The model under review builds one solid part; all positions refer to its coordinate system, in mm. Give positions to 0.01 mm unless a question says otherwise; leave off trailing zeros. Loops run counter-clockwise (first coordinate to the right, second up) from the corner with the lowest first, then second, coordinate; pieces in that order, holes last. Notation, with made-up numbers: (15.25, 22) - (69.25, 22) arc R13 ccw to (69.25, 47) - close; hole circle Ø3 at (47.25, 21). An arc over 180 degrees is marked (long way). Answer as a JSON object with one key per item and string values.
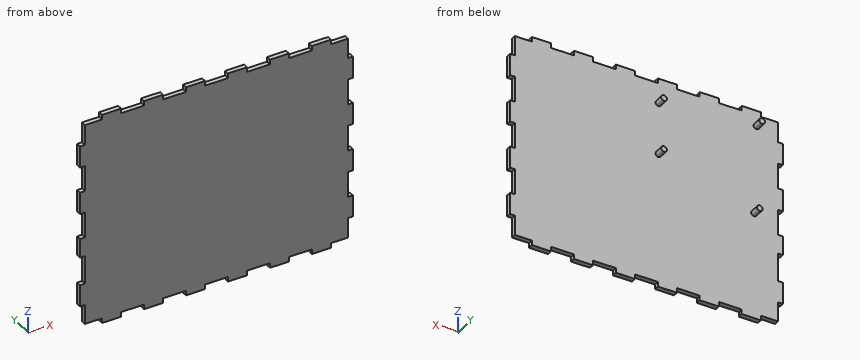
from build123d import *

# Parameters (mm, degrees)
SKETCH1_W           = 144.78
SKETCH1_H           = 114.3
BOSS_EXTRUDE1_DEPTH = 63.5
SKETCH2_W           = 144.78
SKETCH2_H           = 114.3
CUT_EXTRUDE1_DEPTH  = 60.96
SKETCH3_R           = 1.524
BOSS_EXTRUDE2_DEPTH = 5.08
SKETCH4_OUTSIDE_W   = 183.704
SKETCH4_OUTSIDE_H   = 153.224
CUT_EXTRUDE2_DEPTH  = 2.54
SKETCH6_OUTSIDE_W   = 183.704
SKETCH6_OUTSIDE_H   = 153.224
CUT_EXTRUDE4_DEPTH  = 2.54


with BuildPart() as part:
    # Sketch1 → Boss-Extrude1 (new body)
    with BuildSketch(Plane(origin=(0, 0, 0), x_dir=(1, 0, 0), z_dir=(0, 1, 0))):
        Rectangle(SKETCH1_W, SKETCH1_H)
    extrude(amount=BOSS_EXTRUDE1_DEPTH)

    # Sketch2 → Cut-Extrude1 (cut)
    with BuildSketch(Plane(origin=(0, 63.5, 0), x_dir=(1, 0, 0), z_dir=(0, 1, 0))):
        Rectangle(SKETCH2_W, SKETCH2_H)
    extrude(amount=-CUT_EXTRUDE1_DEPTH, mode=Mode.SUBTRACT)

    # Sketch3 → Boss-Extrude2 (add)
    with BuildSketch(Plane(origin=(0, 2.54, 0), x_dir=(1, 0, 0), z_dir=(0, 1, 0))):
        with Locations(Location((-58.42, -48.585184876, 0), (0, 0, 270))):
            Circle(SKETCH3_R)
        with Locations(Location((-6.35, -43.505184876, 0), (0, 0, 270))):
            Circle(SKETCH3_R)
        with Locations(Location((-6.35, -15.565184876, 0), (0, 0, 270))):
            Circle(SKETCH3_R)
        with Locations(Location((-57.15, -0.325184876, 0), (0, 0, 270))):
            Circle(SKETCH3_R)
    extrude(amount=BOSS_EXTRUDE2_DEPTH)

    # Sketch4 outside → Cut-Extrude2 (cut)
    with BuildSketch(Plane(origin=(0, 2.54, 0), x_dir=(1, 0, 0), z_dir=(0, 1, 0))):
        Rectangle(SKETCH4_OUTSIDE_W, SKETCH4_OUTSIDE_H)
        Polygon((69.85, 54.61), (61.296876225, 54.61), (61.296876225, 57.15), (50.159953148, 57.15), (50.159953148, 54.61), (39.023030071, 54.61), (39.023030071, 57.15), (27.886106994, 57.15), (27.886106994, 54.61), (16.749183917, 54.61), (16.749183917, 57.15), (5.61226084, 57.15), (5.61226084, 54.61), (-5.524662236, 54.61), (-5.524662236, 57.15), (-16.661585313, 57.15), (-16.661585313, 54.61), (-27.79850839, 54.61), (-27.79850839, 57.15), (-38.935431467, 57.15), (-38.935431467, 54.61), (-50.072354544, 54.61), (-50.072354544, 57.15), (-61.209277621, 57.15), (-61.209277621, 54.61), (-69.85, 54.61), (-69.85, 44.653580836), (-72.39, 44.653580836), (-72.39, 31.953580836), (-69.85, 31.953580836), (-69.85, 19.253580836), (-72.39, 19.253580836), (-72.39, 6.553580836), (-69.85, 6.553580836), (-69.85, -6.146419164), (-72.39, -6.146419164), (-72.39, -18.846419164), (-69.85, -18.846419164), (-69.85, -31.546419164), (-72.39, -31.546419164), (-72.39, -44.246419164), (-69.85, -44.246419164), (-69.85, -54.61), (-61.209277621, -54.61), (-61.209277621, -57.15), (-50.072354544, -57.15), (-50.072354544, -54.61), (-38.935431467, -54.61), (-38.935431467, -57.15), (-27.79850839, -57.15), (-27.79850839, -54.61), (-16.661585313, -54.61), (-16.661585313, -57.15), (-5.524662236, -57.15), (-5.524662236, -54.61), (5.61226084, -54.61), (5.61226084, -57.15), (16.749183917, -57.15), (16.749183917, -54.61), (27.886106994, -54.61), (27.886106994, -57.15), (39.023030071, -57.15), (39.023030071, -54.61), (50.159953148, -54.61), (50.159953148, -57.15), (61.296876225, -57.15), (61.296876225, -54.61), (69.85, -54.61), (69.85, -44.45), (72.39, -44.45), (72.39, -31.75), (69.85, -31.75), (69.85, -19.05), (72.39, -19.05), (72.39, -6.35), (69.85, -6.35), (69.85, 6.35), (72.39, 6.35), (72.39, 19.05), (69.85, 19.05), (69.85, 31.75), (72.39, 31.75), (72.39, 44.45), (69.85, 44.45), align=None, mode=Mode.SUBTRACT)
    extrude(amount=-CUT_EXTRUDE2_DEPTH, mode=Mode.SUBTRACT)

    # Sketch6 outside → Cut-Extrude4 (cut)
    with BuildSketch(Plane(origin=(0, 2.54, 0), x_dir=(1, 0, 0), z_dir=(0, 1, 0))):
        Rectangle(SKETCH6_OUTSIDE_W, SKETCH6_OUTSIDE_H)
        Polygon((-69.85, 54.61), (-60.701277621, 54.61), (-60.701277621, 57.15), (-50.580354544, 57.15), (-50.580354544, 54.61), (-38.427431467, 54.61), (-38.427431467, 57.15), (-28.30650839, 57.15), (-28.30650839, 54.61), (-16.153585313, 54.61), (-16.153585313, 57.15), (-6.032662236, 57.15), (-6.032662236, 54.61), (6.12026084, 54.61), (6.12026084, 57.15), (16.241183917, 57.15), (16.241183917, 54.61), (28.394106994, 54.61), (28.394106994, 57.15), (38.515030071, 57.15), (38.515030071, 54.61), (50.667953148, 54.61), (50.667953148, 57.15), (60.788876225, 57.15), (60.788876225, 54.61), (69.85, 54.61), (69.85, 43.942), (72.39, 43.942), (72.39, 32.258), (69.85, 32.258), (69.85, 18.542), (72.39, 18.542), (72.39, 6.858), (69.85, 6.858), (69.85, -6.858), (72.39, -6.858), (72.39, -18.542), (69.85, -18.542), (69.85, -32.258), (72.39, -32.258), (72.39, -43.942), (69.85, -43.942), (69.85, -54.61), (60.788876225, -54.61), (60.788876225, -57.15), (50.667953148, -57.15), (50.667953148, -54.61), (38.515030071, -54.61), (38.515030071, -57.15), (28.394106994, -57.15), (28.394106994, -54.61), (16.241183917, -54.61), (16.241183917, -57.15), (6.12026084, -57.15), (6.12026084, -54.61), (-6.032662236, -54.61), (-6.032662236, -57.15), (-16.153585313, -57.15), (-16.153585313, -54.61), (-28.30650839, -54.61), (-28.30650839, -57.15), (-38.427431467, -57.15), (-38.427431467, -54.61), (-50.580354544, -54.61), (-50.580354544, -57.15), (-60.701277621, -57.15), (-60.701277621, -54.61), (-69.85, -54.61), (-69.85, -43.738419164), (-72.39, -43.738419164), (-72.39, -32.054419164), (-69.85, -32.054419164), (-69.85, -18.338419164), (-72.39, -18.338419164), (-72.39, -6.654419164), (-69.85, -6.654419164), (-69.85, 7.061580836), (-72.39, 7.061580836), (-72.39, 17.357767978), (-69.85, 17.357767978), (-69.85, 32.461580836), (-72.39, 32.461580836), (-72.39, 44.145580836), (-69.85, 44.145580836), align=None, mode=Mode.SUBTRACT)
    extrude(amount=-CUT_EXTRUDE4_DEPTH, mode=Mode.SUBTRACT)


solid = part.part
Q1. To check wall thickness, follow probe 1 along Y at (x, z) = (59.5, -17.5); probe 2 along X at (y, z) = (0.5, 48); probe 3 along Z at (x, y) = (20.5, 1). State the ranges of each line that lie inside material, in increasing order. Write a range as [from, to].
Results:
{"probe 1": "y = [0, 2.54]", "probe 2": "x = [-69.85, 69.85]", "probe 3": "z = [-54.61, 54.61]"}
Q2. Consider section B-B, the plane z = 35.5. State the section outline as (x, y) points, plus the area to 3 significant figures.
Results:
{"outline": "(-72.39, 0) - (72.39, 0) - (72.39, 2.54) - (-72.39, 2.54) - close", "area": "368 mm^2"}
Q3. Clearance check with flat-ended pins moving along their axes: pin 1 Ø0.8 at (x, y) = (70.5, 1.5) entering from +Z; pin 2 Ø3 at (x, y) = (-71, 2) entering from +Z; pin 3 Ø1.5 at (x, z) = (-41.5, -31.5) entering from +Y; pin 4 Ø1 at (x, y) = (-8.5, 6) entering from -Z. State where each tip first meets the part, or that it passes through.
Results:
{"pin 1": "stops at z = 43.94", "pin 2": "stops at z = 54.61", "pin 3": "stops at y = 2.54", "pin 4": "passes through"}
Q4. Consider section A-A, the plane y = 4.75. State the section outline as (x, z) points.
Results:
{"outline": "circle Ø3.05 at (-58.42, 48.59); circle Ø3.05 at (-57.15, 0.33); circle Ø3.05 at (-6.35, 15.57); circle Ø3.05 at (-6.35, 43.51)"}
Q5. Consider section C-C, the plane x = -43. State the section outline as (y, z) points, plus the area to 3 significant figures.
Results:
{"outline": "(0, -54.61) - (2.54, -54.61) - (2.54, 54.61) - (0, 54.61) - close", "area": "277 mm^2"}
